Check sheet for the modelled part. Datum: model origin and axes. Units: mm. A direction names the side the tool comes from. Round coordinates to 2 decimals unless told otherwise and drop trailing zeros. Return JSON: item names as keys, results as strings.
from build123d import *

# Parameters (mm, degrees)
BOSS_EXTRUDE1_DEPTH      = 155
CIRPATTERN4_COUNT        = 4
CIRPATTERN4_COPY_1_DEPTH = 155
CIRPATTERN4_COPY_2_DEPTH = 155
CIRPATTERN4_COPY_3_DEPTH = 155


with BuildPart() as part:
    # Sketch2 → Boss-Extrude1 (new body)
    with BuildSketch(Plane.XY):
        with BuildLine():
            Line((-1.366116524, 2.073223305), (-3.116116524, 3.823223305))
            ThreePointArc((-3.116116524, 3.823223305), (-3.189339828, 4), (-3.116116524, 4.176776695))
            Line((-3.116116524, 4.176776695), (-2.292893219, 5))
            Line((-2.292893219, 5), (-3.094974747, 5))
            Line((-3.094974747, 5), (-3.623223305, 4.471751442))
            ThreePointArc((-3.623223305, 4.471751442), (-3.8, 4.398528137), (-3.976776695, 4.471751442))
            Line((-3.976776695, 4.471751442), (-4.505025253, 5))
            Line((-4.505025253, 5), (-4.75, 5))
            ThreePointArc((-4.75, 5), (-4.845670858, 4.980969883), (-4.926776695, 4.926776695))
            Line((-4.926776695, 4.926776695), (0, 0))
            Line((0, 0), (0, 2))
            Line((0, 2), (-1.189339828, 2))
            ThreePointArc((-1.189339828, 2), (-1.285010686, 2.019030117), (-1.366116524, 2.073223305))
        make_face()
    boss_extrude1 = extrude(amount=BOSS_EXTRUDE1_DEPTH)

    # Mirror1: Boss-Extrude1 across plane
    add(boss_extrude1.mirror(Plane(origin=(0, 0, 155), x_dir=(0, 0, 1), z_dir=(0.707106781, 0.707106781, 0))))

    # CirPattern4: Boss-Extrude1 ×4 about axis
    cirpattern4_axis = Axis((0, 0, 0), (0, 0, 1))
    for i in range(1, CIRPATTERN4_COUNT):
        add(boss_extrude1.rotate(cirpattern4_axis, i * 360 / CIRPATTERN4_COUNT))

    # CirPattern4 copy 1 sketch → CirPattern4 copy 1 (add)
    with BuildSketch(Plane.XY):
        with BuildLine():
            Line((-1.366116524, -2.073223305), (-3.116116524, -3.823223305))
            ThreePointArc((-3.116116524, -3.823223305), (-3.189339828, -4), (-3.116116524, -4.176776695))
            Line((-3.116116524, -4.176776695), (-2.292893219, -5))
            Line((-2.292893219, -5), (-3.094974747, -5))
            Line((-3.094974747, -5), (-3.623223305, -4.471751442))
            ThreePointArc((-3.623223305, -4.471751442), (-3.8, -4.398528137), (-3.976776695, -4.471751442))
            Line((-3.976776695, -4.471751442), (-4.505025253, -5))
            Line((-4.505025253, -5), (-4.75, -5))
            ThreePointArc((-4.75, -5), (-4.845670858, -4.980969883), (-4.926776695, -4.926776695))
            Line((-4.926776695, -4.926776695), (0, 0))
            Line((0, 0), (0, -2))
            Line((0, -2), (-1.189339828, -2))
            ThreePointArc((-1.189339828, -2), (-1.285010686, -2.019030117), (-1.366116524, -2.073223305))
        make_face()
    extrude(amount=CIRPATTERN4_COPY_1_DEPTH)

    # CirPattern4 copy 2 sketch → CirPattern4 copy 2 (add)
    with BuildSketch(Plane(origin=(0, 0, 0), x_dir=(0, 1, 0), z_dir=(0, 0, 1))):
        with BuildLine():
            Line((-1.366116524, -2.073223305), (-3.116116524, -3.823223305))
            ThreePointArc((-3.116116524, -3.823223305), (-3.189339828, -4), (-3.116116524, -4.176776695))
            Line((-3.116116524, -4.176776695), (-2.292893219, -5))
            Line((-2.292893219, -5), (-3.094974747, -5))
            Line((-3.094974747, -5), (-3.623223305, -4.471751442))
            ThreePointArc((-3.623223305, -4.471751442), (-3.8, -4.398528137), (-3.976776695, -4.471751442))
            Line((-3.976776695, -4.471751442), (-4.505025253, -5))
            Line((-4.505025253, -5), (-4.75, -5))
            ThreePointArc((-4.75, -5), (-4.845670858, -4.980969883), (-4.926776695, -4.926776695))
            Line((-4.926776695, -4.926776695), (0, 0))
            Line((0, 0), (0, -2))
            Line((0, -2), (-1.189339828, -2))
            ThreePointArc((-1.189339828, -2), (-1.285010686, -2.019030117), (-1.366116524, -2.073223305))
        make_face()
    extrude(amount=CIRPATTERN4_COPY_2_DEPTH)

    # CirPattern4 copy 3 sketch → CirPattern4 copy 3 (add)
    with BuildSketch(Plane(origin=(0, 0, 0), x_dir=(-1, 0, 0), z_dir=(0, 0, 1))):
        with BuildLine():
            Line((-1.366116524, -2.073223305), (-3.116116524, -3.823223305))
            ThreePointArc((-3.116116524, -3.823223305), (-3.189339828, -4), (-3.116116524, -4.176776695))
            Line((-3.116116524, -4.176776695), (-2.292893219, -5))
            Line((-2.292893219, -5), (-3.094974747, -5))
            Line((-3.094974747, -5), (-3.623223305, -4.471751442))
            ThreePointArc((-3.623223305, -4.471751442), (-3.8, -4.398528137), (-3.976776695, -4.471751442))
            Line((-3.976776695, -4.471751442), (-4.505025253, -5))
            Line((-4.505025253, -5), (-4.75, -5))
            ThreePointArc((-4.75, -5), (-4.845670858, -4.980969883), (-4.926776695, -4.926776695))
            Line((-4.926776695, -4.926776695), (0, 0))
            Line((0, 0), (0, -2))
            Line((0, -2), (-1.189339828, -2))
            ThreePointArc((-1.189339828, -2), (-1.285010686, -2.019030117), (-1.366116524, -2.073223305))
        make_face()
    extrude(amount=CIRPATTERN4_COPY_3_DEPTH)


solid = part.part
Q1. Tool access check on faces 4 (the face through (0, 0, 0)), 5 (the face through (0, 2, 76)), 6 (the face through (2, 0, 76)). Record the directions out of +Z, -Z, +X, -X, +Y, -Y that give a thin tool (end or side, any length) a straight path to the whole face; none if there is none.
Answer key:
{"face 4": "-Z, +X, -X, +Y, -Y", "face 5": "+Z, -Z, +Y", "face 6": "+Z, -Z, +X"}
Q2. Depth check by flat-ended pin: P1, Ø1, axis at y = -3.5, z = 40.5, coming from the +X side; P2, Ø1.2, axis at y = -0.5, z = 65.5, coming from the +X side; P3, Ø0.7, axis at x = 0.5, z = 71.5, coming from the +Y side; P4, Ø2.5, axis at y = 0.5, z = 77, coming from the -X side. Enter the tip coordinate at first touch or a pass-through.
Answer key:
{"P1": "stops at x = 5", "P2": "stops at x = 2", "P3": "stops at y = 2", "P4": "stops at x = -2.46"}
Q3. Draft check along X on faces 1 (the face through (0, -2, 76)), 2 (the face through (-2, 0, 76)), 3 (the face through (0, 0, 155)). Enter one of: released by +X, released by -X, zero draft, split by the parting line, or undercut.
Answer key:
{"face 1": "undercut", "face 2": "released by -X", "face 3": "zero draft"}
Q4. Scan lines: probe 1 along X at (y, z) = (-2.5, 111); probe 2 along X at (y, z) = (-2.75, 64.5); probe 3 along Y at (x, z) = (3, 139). Record each from-to range of solid material in increasing order. Write a range as [from, to].
Answer key:
{"probe 1": "x = [-5, -4.79], [-3.21, -1.79], [1.79, 3.21], [4.79, 5]", "probe 2": "x = [-5, -4.54], [-3.46, -2.04], [2.04, 3.46], [4.54, 5]", "probe 3": "y = [-5, -4.29], [-3.71, -2.29], [2.29, 3.71], [4.29, 5]"}
